```python
from build123d import *

# Parameters (mm, degrees)
BOSS_EXTRUDE1_DEPTH = 3.175
BOSS_EXTRUDE2_DEPTH = 3.175
FILLET1_R           = 0.635


with BuildPart() as part:
    # Sketch1 → Boss-Extrude1 (new body)
    with BuildSketch(Plane(origin=(0, 0, 0), x_dir=(1, 0, 0), z_dir=(0, 1, 0))):
        with BuildLine():
            Line((-157.73462252, 34.703486642), (-119.73462252, 34.703486642))
            ThreePointArc((-119.73462252, 34.703486642), (-116.199088614, 36.167952736), (-114.73462252, 39.703486642))
            Line((-114.73462252, 39.703486642), (-114.73462252, 63.703486642))
            ThreePointArc((-114.73462252, 63.703486642), (-116.199088614, 67.239020548), (-119.73462252, 68.703486642))
            Line((-119.73462252, 68.703486642), (-157.73462252, 68.703486642))
            ThreePointArc((-157.73462252, 68.703486642), (-161.270156426, 67.239020548), (-162.73462252, 63.703486642))
            Line((-162.73462252, 63.703486642), (-162.73462252, 39.703486642))
            ThreePointArc((-162.73462252, 39.703486642), (-161.270156426, 36.167952736), (-157.73462252, 34.703486642))
        make_face()
        with BuildLine():
            Line((-134.5215585, 44.703486642), (-142.94768654, 44.703486642))
            ThreePointArc((-142.94768654, 44.703486642), (-146.073167891, 42.667101856), (-149.73462252, 41.953486642))
            ThreePointArc((-149.73462252, 41.953486642), (-159.48462252, 51.703486642), (-149.73462252, 61.453486642))
            ThreePointArc((-149.73462252, 61.453486642), (-146.073167891, 60.739871428), (-142.94768654, 58.703486642))
            Line((-142.94768654, 58.703486642), (-134.5215585, 58.703486642))
            ThreePointArc((-134.5215585, 58.703486642), (-131.396077149, 60.739871428), (-127.73462252, 61.453486642))
            ThreePointArc((-127.73462252, 61.453486642), (-117.98462252, 51.703486642), (-127.73462252, 41.953486642))
            ThreePointArc((-127.73462252, 41.953486642), (-131.396077149, 42.667101856), (-134.5215585, 44.703486642))
        make_face(mode=Mode.SUBTRACT)
        with BuildLine():
            ThreePointArc((-121.23462252, 37.353486642), (-119.63462252, 38.953486642), (-121.23462252, 40.553486642))
            ThreePointArc((-121.23462252, 40.553486642), (-122.83462252, 38.953486642), (-121.23462252, 37.353486642))
        make_face(mode=Mode.SUBTRACT)
        with BuildLine():
            ThreePointArc((-156.23462252, 37.353486642), (-154.63462252, 38.953486642), (-156.23462252, 40.553486642))
            ThreePointArc((-156.23462252, 40.553486642), (-157.83462252, 38.953486642), (-156.23462252, 37.353486642))
        make_face(mode=Mode.SUBTRACT)
        with BuildLine():
            ThreePointArc((-156.23462252, 62.853486642), (-154.63462252, 64.453486642), (-156.23462252, 66.053486642))
            ThreePointArc((-156.23462252, 66.053486642), (-157.83462252, 64.453486642), (-156.23462252, 62.853486642))
        make_face(mode=Mode.SUBTRACT)
        with BuildLine():
            ThreePointArc((-121.23462252, 62.853486642), (-119.63462252, 64.453486642), (-121.23462252, 66.053486642))
            ThreePointArc((-121.23462252, 66.053486642), (-122.83462252, 64.453486642), (-121.23462252, 62.853486642))
        make_face(mode=Mode.SUBTRACT)
    extrude(amount=BOSS_EXTRUDE1_DEPTH)

    # Sketch2 → Boss-Extrude2 (add)
    with BuildSketch(Plane.XZ):
        with BuildLine():
            Line((-169.08462252, -29.024879137), (-169.08462252, -74.382094147))
            ThreePointArc((-169.08462252, -74.382094147), (-164.359232711, -70.120144783), (-158.159635896, -68.685390257))
            ThreePointArc((-158.159635896, -68.685390257), (-161.417357026, -67.085419013), (-162.73462252, -63.703486642))
            Line((-162.73462252, -63.703486642), (-162.73462252, -39.703486642))
            ThreePointArc((-162.73462252, -39.703486642), (-161.417357026, -36.321554271), (-158.159635896, -34.721583027))
            ThreePointArc((-158.159635896, -34.721583027), (-164.359232711, -33.286828501), (-169.08462252, -29.024879137))
        make_face()
    extrude(amount=-BOSS_EXTRUDE2_DEPTH)

    # Fillet1
    fillet1_edges = [part.edges().sort_by_distance(p)[0] for p in [
        (-169.08462252, 1.5875, -74.382094147),
        (-169.08462252, 1.5875, -29.024879137),
    ]]
    fillet(fillet1_edges, radius=FILLET1_R)


solid = part.part
```
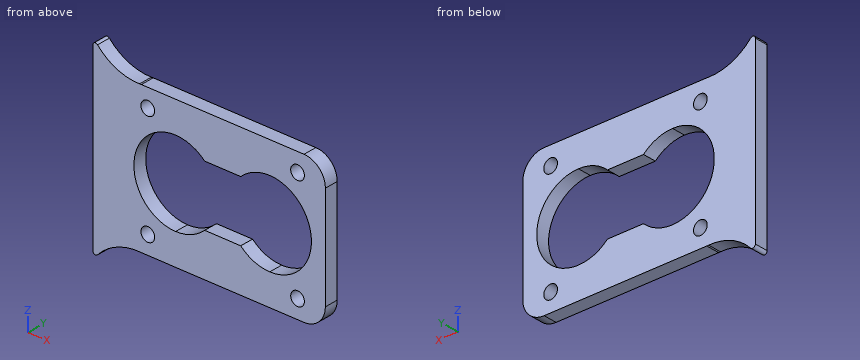
CAD build for the part. Positions are in the model's coordinates, mm. Round coordinates to 2 decimals unless told otherwise and drop trailing zeros. Write each loop counter-clockwise with the first axis right and the second up, starting at its lowest first coordinate (ties: lowest second). Pieces come first, ordered by that corner, then holes. Notation, with made-up numbers: M -11.5,-7.75 L 10.5,-7.75 A24 ccw 10.5,7.25 Z; hole C 72.5,62 d8. An arc over 180 degrees is marked long. One line per question, with ' | ' between items.
1. Probe L1, parallel to X at y = 0.7, z = -51.5; L2, parallel to Z at x = -127.5, y = 0.8; L3, parallel to X at y = 1.7, z = -37.5. List the from-to ranges inside material, lowest first. Write a range as from..to.
Working result:
L1: -169.08..-159.48, -117.99..-114.73 | L2: -68.7..-61.45, -41.96..-34.7 | L3: -169.08..-156.9, -155.57..-121.9, -120.57..-115.25
2. Cut at D-D on z = -70. Write the cut outline in (x, y) (3 decimals), and give its area (3 significant figures).
Working result:
outline: M -169.085,0 L -164.123,0 L -164.123,3.175 L -169.085,3.175 Z | area: 15.8 mm2
3. Cut at B-B on z = -54.5. Write the cut outline in (x, y) (3 decimals).
Working result:
outline: M -169.085,0 L -159.075,0 L -159.075,3.175 L -169.085,3.175 Z; M -118.394,0 L -114.735,0 L -114.735,3.175 L -118.394,3.175 Z
4. Cut at C-C on y = 2.35. Write the cut outline in (x, z) (3 decimals), and give its area (3 significant figures).
Working result:
outline: M -169.085,-72.517 A0.635 ccw -167.975,-72.939 A12.7 cw -158.16,-68.685 A5 ccw -157.735,-68.703 L -119.735,-68.703 A5 ccw -114.735,-63.703 L -114.735,-39.703 A5 ccw -119.735,-34.703 L -157.735,-34.703 A5 ccw -158.16,-34.722 A12.7 cw -167.975,-30.468 A0.635 ccw -169.085,-30.89 Z; hole C -156.235,-64.453 d3.2; hole C -156.235,-38.953 d3.2; hole M -142.948,-58.703 L -134.522,-58.703 A9.75 ccw long -134.522,-44.703 L -142.948,-44.703 A9.75 ccw long Z; hole C -121.235,-64.453 d3.2; hole C -121.235,-38.953 d3.2 | area: 1,180 mm2
5. Pin check, flat tips, straight feed: pin 1 Ø1.6 at (x, y) = (-145, 1.5) entering from -Z; pin 2 Ø1 at (y, z) = (2, -67) entering from +X; pin 3 Ø1.9 at (x, z) = (-156.23, -64.45) entering from -Y; pin 4 Ø1.6 at (x, y) = (-137.5, 1) entering from +Z. Stop position of each tip, or through.
Working result:
pin 1: z = -68.7 | pin 2: x = -115.59 | pin 3: through | pin 4: z = -34.7
6. Cut at A-A on x = -145. Write the cut outline in (y, z) (3 decimals), and give its area (3 significant figures).
Working result:
outline: M 0,-68.703 L 3.175,-68.703 L 3.175,-60.227 L 0,-60.227 Z; M 0,-43.18 L 3.175,-43.18 L 3.175,-34.703 L 0,-34.703 Z | area: 53.8 mm2
